```python
from build123d import *

# Parameters (mm, degrees)
SKETCH1_W                 = 76.2
SKETCH1_H                 = 107.95
BOSS_EXTRUDE1_DEPTH       = 6.35
SKETCH2_R                 = 1.7526
SKETCH2_W                 = 12.7
SKETCH2_H                 = 6.35
SKETCH2_W_2               = 25.4
CUT_EXTRUDE1_DEPTH        = 6.35
F_6_CLEARANCE_HOLE1_D     = 3.7973
F_6_CLEARANCE_HOLE1_DEPTH = 6.35
F_6_CLEARANCE_HOLE1_TIP   = 1.140824014


with BuildPart() as part:
    # Sketch1 → Boss-Extrude1 (new body)
    with BuildSketch(Plane(origin=(0, 0, 0), x_dir=(1, 0, 0), z_dir=(0, 1, 0))):
        Rectangle(SKETCH1_W, SKETCH1_H)
    extrude(amount=BOSS_EXTRUDE1_DEPTH)

    # Sketch2 → Cut-Extrude1 (cut)
    with BuildSketch(Plane(origin=(0, 6.35, 0), x_dir=(1, 0, 0), z_dir=(0, 1, 0))):
        with Locations(Location((-19.05, 50.8, 0), (0, 0, 270))):
            Circle(SKETCH2_R)
        with Locations(Location((19.05, 50.8, 0), (0, 0, 270))):
            Circle(SKETCH2_R)
        with Locations(Location((19.05, -50.8, 0), (0, 0, 90))):
            Circle(SKETCH2_R)
        with Locations(Location((-19.05, -50.8, 0), (0, 0, 90))):
            Circle(SKETCH2_R)
        with Locations((-31.75, 50.8)):
            Rectangle(SKETCH2_W, SKETCH2_H)
        with Locations((0, 50.8)):
            Rectangle(SKETCH2_W_2, SKETCH2_H)
        with Locations((31.75, 50.8)):
            Rectangle(SKETCH2_W, SKETCH2_H)
        with Locations((31.75, -50.8)):
            Rectangle(SKETCH2_W, SKETCH2_H)
        with Locations((0, -50.8)):
            Rectangle(SKETCH2_W_2, SKETCH2_H)
        with Locations((-31.75, -50.8)):
            Rectangle(SKETCH2_W, SKETCH2_H)
    extrude(amount=-CUT_EXTRUDE1_DEPTH, mode=Mode.SUBTRACT)

    # #6 Clearance Hole1
    with Locations(Plane(origin=(0, 6.35, 0), x_dir=(1, 0, 0), z_dir=(0, 1, 0))):
        with Locations((-19.05, 50.8), (19.05, 50.8), (-19.05, -50.8), (19.05, -50.8)):
            Hole(F_6_CLEARANCE_HOLE1_D / 2, depth=F_6_CLEARANCE_HOLE1_DEPTH)
            with Locations((0, 0, -(F_6_CLEARANCE_HOLE1_DEPTH + F_6_CLEARANCE_HOLE1_TIP / 2))):  # 118° drill point
                Cone(0, F_6_CLEARANCE_HOLE1_D / 2, F_6_CLEARANCE_HOLE1_TIP, mode=Mode.SUBTRACT)


solid = part.part
```
Geometry: final body of the model. Coordinates: model frame, mm. A direction names the side the tool comes from. Give positions to 0.01 mm unless a question says otherwise; leave off trailing zeros. Order: outer loops, then holes, each group sorted by start corner. A loop starts at its lowest first (then second) coordinate and runs counter-clockwise, first axis right, second up. Notation, with made-up numbers: M 2.5,-4 L 30.5,-4 A27 ccw 30.5,24 Z; hole C 8.5,0 d3. An arc over 180 degrees is marked long. Answer as CSV lines item,"result". Start each with the question number.
1) First-contact query: P1, Ø1.9, axis at x = -4, y = 2, coming from the +Z side (3 decimals); P2, Ø1.9, axis at y = 2.5, z = 51, coming from the -X side; P3, Ø1.9, axis at x = -0.5, y = 2.5, coming from the -Z side (3 decimals); P4, Ø3, axis at x = -19.05, z = 50.8, coming from the -Y side. Flat tips, straight axial feed; report the tip coordinate or a pass-through.
2) Set-up query: faces 1 (the flat face through (0, 3, -47.625)), 2 (the flat face through (0, 3, 47.625)), 3 (the flat face through (32, 3, -47.625)), 4 (the flat face through (32, 3, 47.625)). Return all of +Z, -Z, +X, -X, +Y, -Y with unobstructed straight access to the full face (end or side cutting, diameter ignored); none if empty.
3) Cut plane D-D (x = 30). Output: boundary loops of the cut face in (y, z) (3 decimals), then the cut area to 3 significant figures.
4) Cut plane C-C (z = 50.8). Output: boundary loops of the cut face in (x, y).
5) Cut plane A-A (x = -19.05). Output: boundary loops of the cut face in (y, z) (3 decimals), then the cut area to 3 significant figures.
6) Cut plane B-B (y = 4). Output: boundary loops of the cut face in (x, z) (3 decimals).
7) Line query: line 1 (X direction, y = 4, z = 50.8); line 2 (Z direction, x = 19.05, y = 4.25) (3 decimals); line 3 (Z direction, x = 18, y = 5) (3 decimals). Output: solid intervals per line, ascending. Write a range as from..to.
8) Mould query, pull axis Z, two halves, no side actions, for faces 5 (the flat face through (-32, 3, -47.625)), 6 (the cylindrical face through (19.462, 3.131, 52.654)), 7 (the flat face through (-32, 3, 47.625)). Classes: +Z half, -Z half, draft (parallel to the pull), parting line (faces both ways), or undercut.
Findings below:
1,P1,"stops at z = 47.625"
1,P2,"stops at x = -25.4"
1,P3,"stops at z = -47.625"
1,P4,"passes through"
2,face 1,"-Z, +Y, -Y"
2,face 2,"+Z, +Y, -Y"
2,face 3,"-Z, +X, +Y, -Y"
2,face 4,"+Z, +X, +Y, -Y"
3,outline,"M 0,-47.625 L 6.35,-47.625 L 6.35,47.625 L 0,47.625 Z"
3,area,"605 mm²"
4,outline,"M -25.4,0 L -20.95,0 L -20.95,6.35 L -25.4,6.35 Z; M -17.15,0 L -12.7,0 L -12.7,6.35 L -17.15,6.35 Z; M 12.7,0 L 17.15,0 L 17.15,6.35 L 12.7,6.35 Z; M 20.95,0 L 25.4,0 L 25.4,6.35 L 20.95,6.35 Z"
5,outline,"M 0,-53.975 L 6.35,-53.975 L 6.35,-52.699 L 0,-52.699 Z; M 0,-48.901 L 6.35,-48.901 L 6.35,48.901 L 0,48.901 Z; M 0,52.699 L 6.35,52.699 L 6.35,53.975 L 0,53.975 Z"
5,area,"637 mm²"
6,outline,"M -38.1,-47.625 L -25.4,-47.625 L -25.4,-53.975 L -12.7,-53.975 L -12.7,-47.625 L 12.7,-47.625 L 12.7,-53.975 L 25.4,-53.975 L 25.4,-47.625 L 38.1,-47.625 L 38.1,47.625 L 25.4,47.625 L 25.4,53.975 L 12.7,53.975 L 12.7,47.625 L -12.7,47.625 L -12.7,53.975 L -25.4,53.975 L -25.4,47.625 L -38.1,47.625 Z; hole C -19.05,-50.8 d3.797; hole C -19.05,50.8 d3.797; hole C 19.05,-50.8 d3.797; hole C 19.05,50.8 d3.797"
7,line 1,"x = -25.4..-20.95, -17.15..-12.7, 12.7..17.15, 20.95..25.4"
7,line 2,"z = -53.975..-52.699, -48.901..48.901, 52.699..53.975"
7,line 3,"z = -53.975..-52.382, -49.218..49.218, 52.382..53.975"
8,face 5,"-Z half"
8,face 6,"undercut"
8,face 7,"+Z half"
